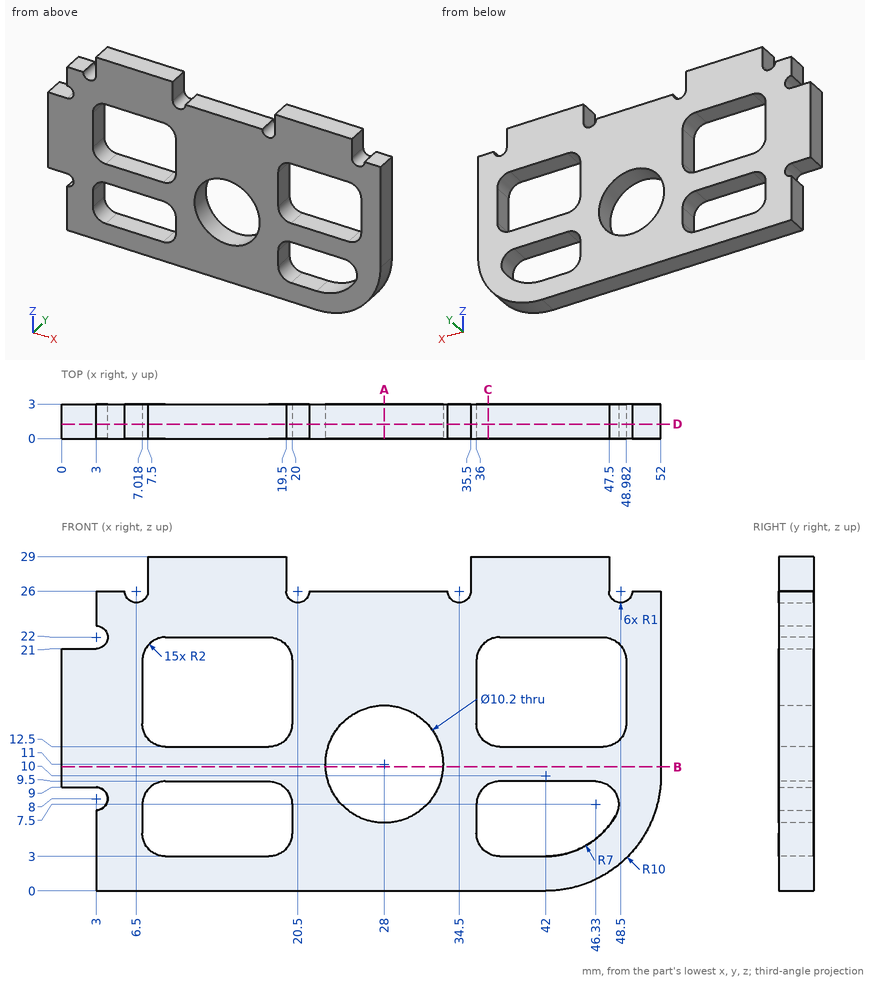
Source: three-view drawing plus pictorial views. Frame: mm from the lowest corner of the part. Give positions to 0.01 mm unless a question says otherwise; leave off trailing zeros. Order: outer loops, then holes, each group sorted by start corner. A loop starts at its lowest first (then second) coordinate and runs counter-clockwise, first axis right, second up. Notation, with made-up numbers: (3, 66) - (19, 66) arc R28 cw to (19, 101) - close; hole circle Ø6 at (22, -32). An arc over 180 degrees is marked (long way). Put each result on its own line as item: value.
Item 1: Section query C-C, the plane x = 37. Return loops of the section in (y, z), then the cut area to 3 significant figures.
Found:
outline: (0, 0) - (3, 0) - (3, 3.27) - (0, 3.27) - close; (0, 9.23) - (3, 9.23) - (3, 12.77) - (0, 12.77) - close; (0, 21.73) - (3, 21.73) - (3, 29) - (0, 29) - close
area: 42.2 mm^2
Item 2: Section query B-B, the plane z = 10.75. Return loops of the section in (x, y).
Found:
outline: (0, 0) - (22.91, 0) - (22.91, 3) - (0, 3) - close; (33.09, 0) - (52, 0) - (52, 3) - (33.09, 3) - close
Item 3: Section query A-A, the plane x = 28. Return loops of the section in (y, z).
Found:
outline: (0, 0) - (3, 0) - (3, 5.9) - (0, 5.9) - close; (0, 16.1) - (3, 16.1) - (3, 26) - (0, 26) - close
Item 4: Ray query, L1, parallel to X at y = 0.25, z = 20; L2, parallel to X at y = 1.55, z = 11; L3, parallel to Z at x = 10.5, y = 1.9. Return the intervals inside material, ascending. Write a range as from..to.
Found:
L1: x = 0..7.02, 20..36, 48.98..52
L2: x = 0..22.9, 33.1..52
L3: z = 0..3, 9.5..12.5, 22..29
Item 5: Section query D-D, the plane y = 1.25. Count the separate pieces of the cut face and the enclosed holes in it, then the cut area to 3 significant figures.
Found:
separate pieces: 1
enclosed holes: 5
area: 878 mm^2
Item 6: Contact query for flat-ended pins moving along their axis: pin 1 (0.9 mm diameter, centred on y = 1, z = 2, fed in from -X); pin 2 (1.2 mm diameter, centred on x = 51, y = 1, fed in from +Z); pin 3 (0.9 mm diameter, centred on y = 2, z = 27.5, fed in from +X). Output: stop coordinate, or through.
Found:
pin 1: stops at x = 3
pin 2: stops at z = 26
pin 3: stops at x = 47.5
